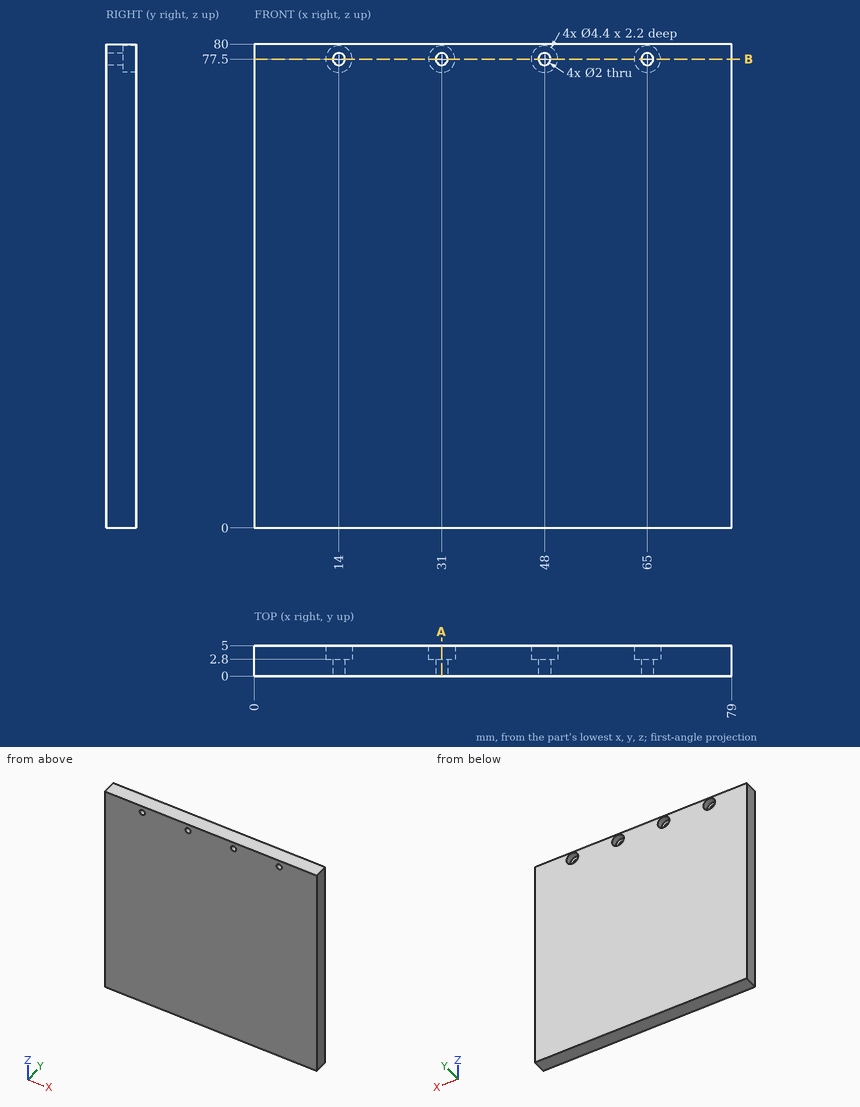
Print and shaded views of the part. All mm, measured from the part's lowest x, y and z. Round coordinates to 2 decimals unless told otherwise and drop trailing zeros. Write each loop counter-clockwise with the first axis right and the second up, starting at its lowest first coordinate (ties: lowest second). Pieces come first, ordered by that corner, then holes. Notation, with made-up numbers: (-17, -1) - (-8, -1) arc R19 ccw to (-8, 4) - close; hole circle Ø2 at (39, 17). An arc over 180 degrees is marked (long way). One line per question, with ' | ' between items.
1. Drop flat-ended pins along their axis: pin 1 Ø1 at (y, z) = (2, 62.5) entering from -X; pin 2 Ø3.5 at (x, z) = (65, 77.5) entering from +Y; pin 3 Ø1.8 at (x, z) = (14, 77.5) entering from +Y. Give the stop position or say it passes through.
Results are:
pin 1: x = 0 | pin 2: y = 2.8 | pin 3: through
2. Drill centre lines: line 1 along X through (y, z) = (4.2, 77.5); line 2 along X through (y, z) = (1.5, 77.5); line 3 along Z through (x, y) = (48, 3.65). Where is each one in solid material? Low to high. Write a range as from..to.
Results are:
line 1: 0..11.8, 16.2..28.8, 33.2..45.8, 50.2..62.8, 67.2..79 | line 2: 0..13, 15..30, 32..47, 49..64, 66..79 | line 3: 0..75.3, 79.7..80
3. Band-saw the part on B-B, the plane z = 77.5. Give the number of separate pieces and of enclosed holes in the cut face, and give its area (3 significant figures).
Results are:
separate pieces: 5 | enclosed holes: 0 | area: 334 mm^2
4. Band-saw the part on A-A, the plane x = 31. Write the cut outline in (y, z).
Results are:
outline: (0, 0) - (5, 0) - (5, 75.3) - (2.8, 75.3) - (2.8, 76.5) - (0, 76.5) - close; (0, 78.5) - (2.8, 78.5) - (2.8, 79.7) - (5, 79.7) - (5, 80) - (0, 80) - close
